Read the model definition and answer for the solid it produces. Units are mm, in the model's axes. Face numbers are marked on the shaded views. A direction names the side the tool comes from. Coordinates: 2 decimals unless noted, no trailing zeros. Write each loop counter-clockwise with the first axis right and the second up, starting at its lowest first coordinate (ties: lowest second). Pieces come first, ordered by that corner, then holes. Notation, with made-up numbers: (5.25, -6.5) -> (20.25, -6.5) arc R24 cw to (20.25, 6.5) -> close; hole circle Ø1 at (42, 54). An arc over 180 degrees is marked (long way). Answer as a JSON object with one key per item and string values. Group by question number.
(1) Find section D-D (x = 21). Give the vertices of the cut face in (y, z), then the cut area to 3 significant figures.
(2) Straight lines are drawn through the part: L1, parallel to X at y = -15.75, z = 0; L2, parallel to X at y = -13.75, z = 19; L3, parallel to Z at x = 0, y = -15.9. For each, find the intervals that lie inside material, in ascending order.
(3) Find section C-C (y = -8.25). Give the vertices of the cut face in (x, z).
(4) Flat-ended cylindrical pins translate along their axes: P1, Ø1.5, axis at x = 8, y = -8, coming from the -Z side; P2, Ø4, axis at x = -17.5, y = -20, coming from the +Z side; P3, Ø10, axis at x = -1, y = -8, coming from the +Z side; P4, Ø8, axis at x = -15, y = -2.5, coming from the +Z side. Find the tip coordinate at first contact, or state that the pin passes through.
(5) Which of the six approach directions +Z, -Z, +X, -X, +Y, -Y give full straight-line access (tool end or side, diameter ignored) to the marked faces 1 and 2?
(6) Find section A-A (z = 0). Give the vertices of the cut face in (x, y), then the cut area to 3 significant figures.
(7) For a pull along X with two mould halves and no side action, classify the marked faces 3, 4 and 5 as +X half, -X half, draft (parallel to the pull), parting line (faces both ways), or undercut.
(8) Find section B-B (x = 0). Give the vertices of the cut face in (y, z), then the cut area to 3 significant figures.
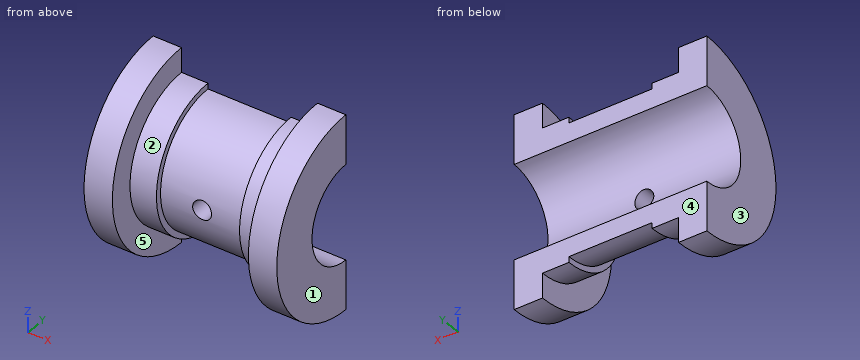
from build123d import *

# Parameters (mm, degrees)
REVOLVE3_ANGLE           = 180
CUT_EXTRUDE1_DEPTH       = 52
F_6_0_6_DIAMETER_HOLE1_D = 5


with BuildPart() as part:
    # Sketch2 → Revolve3 (revolve)
    with BuildSketch(Plane(origin=(0, 0, 0), x_dir=(1, 0, 0), z_dir=(0, 1, 0))):
        Polygon((25.5, 0), (-25.5, 0), (-25.5, 25.5), (-18, 25.5), (-18, 19), (-11, 19), (-11, 17.5), (11, 17.5), (11, 19), (18, 19), (18, 25.5), (25.5, 25.5), align=None)
    revolve(axis=Axis((25.5, 0, 0), (-1, 0, 0)), revolution_arc=REVOLVE3_ANGLE)

    # Sketch3 → Cut-Extrude1 (cut, through all)
    with BuildSketch(Plane.ZY.offset(25.5)):
        with BuildLine():
            Line((12.5, 0), (-12.5, 0))
            ThreePointArc((-12.5, 0), (0, -12.5), (12.5, 0))
        make_face()
    extrude(amount=-CUT_EXTRUDE1_DEPTH, mode=Mode.SUBTRACT)

    # Ø6.0 (6) Diameter Hole1 (through all)
    with Locations(Plane(origin=(0, -17.5, 0), x_dir=(0, 0, -1), z_dir=(0, -1, 0))):
        with Locations((0, 0)):
            Hole(F_6_0_6_DIAMETER_HOLE1_D / 2)


solid = part.part
Results below:
{
 "1": {"outline": "(0, -25.5) -> (0, -12.5) arc R12.5 cw to (0, 12.5) -> (0, 25.5) arc R25.5 ccw to start", "area": "776 mm2"},
 "2": {"L1": "x = -25.5 to -2.5, 2.5 to 25.5", "L2": "x = -25.5 to -18, 18 to 25.5", "L3": "z = -7.31 to -2.5, 2.5 to 7.31"},
 "3": {"outline": "(-25.5, -24.13) -> (-18, -24.13) -> (-18, -17.12) -> (-11, -17.12) -> (-11, -15.43) -> (11, -15.43) -> (11, -17.12) -> (18, -17.12) -> (18, -24.13) -> (25.5, -24.13) -> (25.5, -9.39) -> (-25.5, -9.39) -> close; (-25.5, 9.39) -> (25.5, 9.39) -> (25.5, 24.13) -> (18, 24.13) -> (18, 17.12) -> (11, 17.12) -> (11, 15.43) -> (-11, 15.43) -> (-11, 17.12) -> (-18, 17.12) -> (-18, 24.13) -> (-25.5, 24.13) -> close"},
 "4": {"P1": "stops at z = -15.93", "P2": "stops at z = 18", "P3": "stops at z = 17.24", "P4": "stops at z = 25.5"},
 "5": {"face 1": "+Z, -Z, +X, +Y, -Y", "face 2": "-Y"},
 "6": {"outline": "(-25.5, -25.5) -> (-18, -25.5) -> (-18, -19) -> (-11, -19) -> (-11, -17.5) -> (-2.5, -17.5) -> (-2.5, -12.5) -> (-25.5, -12.5) -> close; (2.5, -17.5) -> (11, -17.5) -> (11, -19) -> (18, -19) -> (18, -25.5) -> (25.5, -25.5) -> (25.5, -12.5) -> (2.5, -12.5) -> close", "area": "371 mm2"},
 "7": {"face 3": "-X half", "face 4": "draft", "face 5": "undercut"},
 "8": {"outline": "(-17.32, -2.5) arc R17.5 ccw to (0, -17.5) -> (0, -12.5) arc R12.5 cw to (-12.25, -2.5) -> close; (-17.32, 2.5) -> (-12.25, 2.5) arc R12.5 cw to (0, 12.5) -> (0, 17.5) arc R17.5 ccw to start", "area": "210 mm2"}
}
